The listing builds one solid part. Answer for the finished solid, in the listing's coordinates (mm). A direction names the side the tool comes from. Coordinates: 2 decimals unless noted, no trailing zeros. Loops run counter-clockwise (first coordinate to the right, second up) from the corner with the lowest first, then second, coordinate; pieces in that order, holes last. Notation, with made-up numbers: M 26,27 L 39,27 A10 cw 39,33 Z; hole C 49,44.5 d5. An arc over 180 degrees is marked long. Answer as a JSON object with one key per item and string values. Group by question number.
1. Given pin 1 (10 mm diameter, centred on y = 7, z = 7, fed in from -X); pin 2 (1.5 mm diameter, centred on x = -1, z = 19, fed in from +Y), each flat-ended and moving along its own axis, determine where each tip first touches the part or whether it passes through.
2. A cutting plane is placed at B-B on y = 7. Give the vertices of the cut face in (x, z), and give its area (3 significant figures).
3. Straight lines are drawn through the part: L1, parallel to Y at x = -13.7, z = -24; L2, parallel to X at y = 13.75, z = -22; L3, parallel to Y at x = 0.75, z = -12. For each, find the intervals that lie inside material, in ascending order.
4. Determine the mould class of faces 5 (the face through (0, -1, 0)), 6 (the face through (-14, 19, 24)), 7 (the face through (14, 21, 0)) for opening direction Y: released by +Y, released by -Y, zero draft, split by the parting line, or undercut.
5. A cutting plane is placed at D-D on z = 12.5. Give the vertices of the cut face in (x, y).
6. For faces 1 (the face through (-13, 11, -24)), 2 (the face through (-14, 11, 21)), 3 (the face through (-15, 0, -2)), 4 (the face through (-14, 7, 22)), determine the directions among +Z, -Z, +X, -X, +Y, -Y from which every point of the face is accessible in a straight line to the end or side of a thin tool.
7. A cutting plane is placed at A-A on z = 24. Give the vertices of the cut face in (x, y).
8. A cutting plane is placed at C-C on x = -8. Give the vertices of the cut face in (y, z).
from build123d import *

# Parameters (mm, degrees)
SKETCH_1_W          = 2
SKETCH_1_H          = 20
SKETCH_1_W_2        = 30
SKETCH_1_H_2        = 2
EXTRUDE_1_DEPTH     = 28
SKETCH_2_W          = 42
SKETCH_2_H          = 20
CUT_EXTRUDE_1_DEPTH = 39.078865529
CUT_EXTRUDE_3_REACH = 48.098
SKETCH_3_R          = 2


with BuildPart() as part:
    # 草图1 → 凸台-拉伸1 (new, symmetric)
    with BuildSketch(Plane.XY):
        with Locations((-14, 11)):
            Rectangle(SKETCH_1_W, SKETCH_1_H)
        Rectangle(SKETCH_1_W_2, SKETCH_1_H_2)
        with Locations((14, 11)):
            Rectangle(SKETCH_1_W, SKETCH_1_H)
    extrude(amount=EXTRUDE_1_DEPTH, both=True)

    # 草图2 → 切除-拉伸1 (cut, through all)
    with BuildSketch(Plane(origin=(0, 0, 0), x_dir=(0, 0, -1), z_dir=(1, 0, 0))):
        with Locations((0, 11)):
            Rectangle(SKETCH_2_W, SKETCH_2_H)
    extrude(amount=-CUT_EXTRUDE_1_DEPTH, mode=Mode.SUBTRACT)

    # 草图3 → 切除-拉伸3 (cut, up to next)
    with BuildSketch(Plane.ZY.offset(15), mode=Mode.PRIVATE) as cut_extrude_3_sk1:
        with Locations((-24, 17)):
            Circle(SKETCH_3_R)
    cut_extrude_3_tool1 = extrude(cut_extrude_3_sk1.sketch, amount=-CUT_EXTRUDE_3_REACH, mode=Mode.PRIVATE) & part.part
    # 草图3 → 切除-拉伸3 (cut, up to next)
    with BuildSketch(Plane.ZY.offset(15), mode=Mode.PRIVATE) as cut_extrude_3_sk2:
        with Locations((-24, 7)):
            Circle(SKETCH_3_R)
    cut_extrude_3_tool2 = extrude(cut_extrude_3_sk2.sketch, amount=-CUT_EXTRUDE_3_REACH, mode=Mode.PRIVATE) & part.part
    # 草图3 → 切除-拉伸3 (cut, up to next)
    with BuildSketch(Plane.ZY.offset(15), mode=Mode.PRIVATE) as cut_extrude_3_sk3:
        with Locations((24, 7)):
            Circle(SKETCH_3_R)
    cut_extrude_3_tool3 = extrude(cut_extrude_3_sk3.sketch, amount=-CUT_EXTRUDE_3_REACH, mode=Mode.PRIVATE) & part.part
    # 草图3 → 切除-拉伸3 (cut, up to next)
    with BuildSketch(Plane.ZY.offset(15), mode=Mode.PRIVATE) as cut_extrude_3_sk4:
        with Locations((24, 17)):
            Circle(SKETCH_3_R)
    cut_extrude_3_tool4 = extrude(cut_extrude_3_sk4.sketch, amount=-CUT_EXTRUDE_3_REACH, mode=Mode.PRIVATE) & part.part
    add(cut_extrude_3_tool1.solids().sort_by_distance((-15, 17, -24))[0], mode=Mode.SUBTRACT)
    add(cut_extrude_3_tool2.solids().sort_by_distance((-15, 7, -24))[0], mode=Mode.SUBTRACT)
    add(cut_extrude_3_tool3.solids().sort_by_distance((-15, 7, 24))[0], mode=Mode.SUBTRACT)
    add(cut_extrude_3_tool4.solids().sort_by_distance((-15, 17, 24))[0], mode=Mode.SUBTRACT)


solid = part.part
From the geometry:
{
 "1": {"pin 1": "stops at x = 13", "pin 2": "stops at y = 1"},
 "2": {"outline": "M -15,-28 L -13,-28 L -13,-26 L -15,-26 Z; M -15,-22 L -13,-22 L -13,-21 L -15,-21 Z; M -15,21 L -13,21 L -13,22 L -15,22 Z; M -15,26 L -13,26 L -13,28 L -15,28 Z; M 13,-28 L 15,-28 L 15,28 L 13,28 Z", "area": "124 mm²"},
 "3": {"L1": "y = -1 to 5, 9 to 15, 19 to 21", "L2": "x = -15 to -13, 13 to 15", "L3": "y = -1 to 1"},
 "4": {"face 5": "released by -Y", "face 6": "undercut", "face 7": "released by +Y"},
 "5": {"outline": "M -15,-1 L 15,-1 L 15,21 L 13,21 L 13,1 L -15,1 Z"},
 "6": {"face 1": "+Z, -Z, +Y", "face 2": "-X, +Y", "face 3": "+Z, -Z, -X, +Y, -Y", "face 4": "-X"},
 "7": {"outline": "M -15,-1 L 15,-1 L 15,21 L 13,21 L 13,1 L -13,1 L -13,5 L -15,5 Z; M -15,9 L -13,9 L -13,15 L -15,15 Z; M -15,19 L -13,19 L -13,21 L -15,21 Z"},
 "8": {"outline": "M -1,-28 L 1,-28 L 1,28 L -1,28 Z"}
}
